Work out the finished part from the listing and answer in its coordinate system (mm). Face numbers are marked on the shaded views. A direction names the side the tool comes from. Coordinates: 2 decimals unless noted, no trailing zeros. Order: outer loops, then holes, each group sorted by start corner. A loop starts at its lowest first (then second) coordinate and runs counter-clockwise, first axis right, second up.
1. The part is cut by section B-B, the plane y = 22.5. Give the vertices of the cut face in (x, z).
2. The part is cut by section A-A, the plane y = 6. Give the vertices of the cut face in (x, z), then the cut area to 3 significant figures.
3. Determine the mould class of the marked faces 3, 4, 5 and 6 for opening direction X: +X half, -X half, draft (parallel to the pull), parting line (faces both ways), or undercut.
4. Find the intervals of material crossed by probe 1 along Z at (x, y) = (21, 29.5); probe 2 along X at (y, z) = (11.5, 43); probe 3 along Y at (x, z) = (-25.5, -38.5), in increasing order.
5. The part is cut by section C-C, the plane z = -11. Give the vertices of the cut face in (x, y), then the cut area to 3 significant figures.
6. A tool of negligible diameter and unlimited length cuts with its end or side. For the marked faces 1 and 2, from which of +Z, -Z, +X, -X, +Y, -Y can it reach the whole face along a straight path? Write none if from no direction.
7. Flat-ended cylindrical pins translate along their axes: pin 1 Ø1.5 at (y, z) = (22.5, -42.5) entering from -X; pin 2 Ø8 at (x, z) = (11, -43) entering from -Y; pin 3 Ø1.2 at (y, z) = (7.5, 43) entering from +X. Find the tip coordinate at first contact, or state that the pin passes through.
8. The part is cut by section D-D, the plane x = -27.5. Give the vertices of the cut face in (y, z), then the cut area to 3 significant figures.
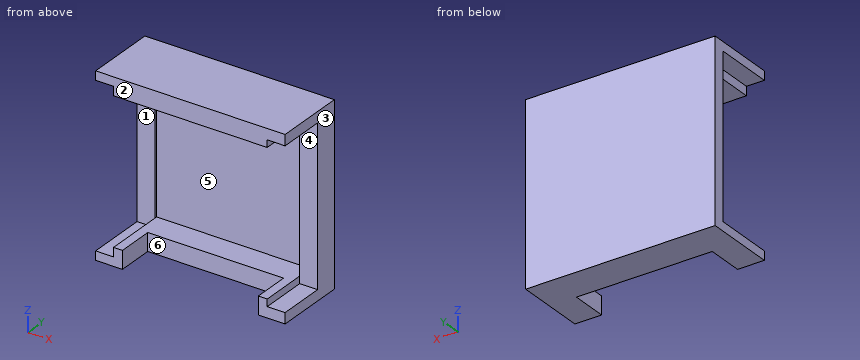
```python
from build123d import *

# Parameters (mm, degrees)
SKETCH1_W               = 106
SKETCH1_H               = 100
BOSS_EXTRUDE1_DEPTH     = 40
SKETCH2_W               = 86
SKETCH2_H               = 80
CUT_EXTRUDE1_DEPTH      = 35
CUT_EXTRUDE2_DEPTH      = 124.838604643
CUT_EXTRUDE2_DEPTH_BACK = 10
SKETCH3_W               = 88
SKETCH3_H               = 26.357936409
SKETCH4_W               = 90
SKETCH4_H               = 33.597569481
CUT_EXTRUDE3_DEPTH      = 10
SKETCH5_W               = 76
SKETCH5_H               = 20.50870907
CUT_EXTRUDE4_DEPTH      = 10


with BuildPart() as part:
    # Sketch1 → Boss-Extrude1 (new body)
    with BuildSketch(Plane(origin=(0, 0, 0), x_dir=(1, 0, 0), z_dir=(0, 1, 0))):
        Rectangle(SKETCH1_W, SKETCH1_H)
    extrude(amount=BOSS_EXTRUDE1_DEPTH)

    # Sketch2 → Cut-Extrude1 (cut)
    with BuildSketch(Plane.XZ):
        Rectangle(SKETCH2_W, SKETCH2_H)
    extrude(amount=-CUT_EXTRUDE1_DEPTH, mode=Mode.SUBTRACT)

    # Sketch3 → Cut-Extrude2 (cut, two sides: drawn at the far end of the back side and taken through both)
    with BuildSketch(Plane(origin=(53, 0, 0), x_dir=(0, 0, -1), z_dir=(1, 0, 0)).offset(-CUT_EXTRUDE2_DEPTH_BACK)):
        with Locations((0, 13.178968205)):
            Rectangle(SKETCH3_W, SKETCH3_H)
    extrude(amount=CUT_EXTRUDE2_DEPTH + CUT_EXTRUDE2_DEPTH_BACK, mode=Mode.SUBTRACT)

    # Sketch4 → Cut-Extrude3 (cut)
    with BuildSketch(Plane.ZY.offset(53)):
        with Locations((0, 16.798784741)):
            Rectangle(SKETCH4_W, SKETCH4_H)
    extrude(amount=-CUT_EXTRUDE3_DEPTH, mode=Mode.SUBTRACT)

    # Sketch5 → Cut-Extrude4 (cut)
    with BuildSketch(Plane(origin=(0, 0, -50), x_dir=(-1, 0, 0), z_dir=(0, 0, -1))):
        with Locations((0, 10.254354535)):
            Rectangle(SKETCH5_W, SKETCH5_H)
    extrude(amount=-CUT_EXTRUDE4_DEPTH, mode=Mode.SUBTRACT)


solid = part.part
```
Geometry says:
1. outline: (-53, -50) - (53, -50) - (53, -44) - (43, -44) - (43, -40) - (-43, -40) - (-43, -45) - (-53, -45) - close; (-53, 45) - (-43, 45) - (-43, 40) - (43, 40) - (43, 44) - (53, 44) - (53, 50) - (-53, 50) - close
2. outline: (-53, -50) - (-38, -50) - (-38, -40) - (-43, -40) - (-43, -45) - (-53, -45) - close; (-53, 45) - (-43, 45) - (-43, 40) - (43, 40) - (43, 44) - (53, 44) - (53, 50) - (-53, 50) - close; (38, -50) - (53, -50) - (53, -44) - (43, -44) - (43, -40) - (38, -40) - close
2. area: 1,180 mm2
3. face 3: +X half
3. face 4: draft
3. face 5: undercut
3. face 6: undercut
4. probe 1: z = -50 to -40, 40 to 50
4. probe 2: x = -43 to 43
4. probe 3: y = 35 to 40
5. outline: (-53, 33.6) - (-43, 33.6) - (-43, 35) - (43, 35) - (43, 26.36) - (53, 26.36) - (53, 40) - (-53, 40) - close
5. area: 630 mm2
6. face 1: -X, -Y
6. face 2: +Z, -Z, +X, -X, -Y
7. pin 1: stops at x = -43
7. pin 2: stops at y = 20.51
7. pin 3: stops at x = 43
8. outline: (0, 40) - (35, 40) - (35, -40) - (20.51, -40) - (20.51, -50) - (40, -50) - (40, 50) - (0, 50) - close
8. area: 995 mm2
